Model file for the job. Use its own axes, mm. Face numbers are marked on the shaded views. A direction names the side the tool comes from. Round coordinates to 2 decimals unless told otherwise and drop trailing zeros. Loops run counter-clockwise (first coordinate to the right, second up) from the corner with the lowest first, then second, coordinate; pieces in that order, holes last. Notation, with made-up numbers: M 42.5,83.25 L 46.5,83.25 A10 ccw 46.5,100.25 Z; hole C 28,-11 d2. An arc over 180 degrees is marked long. Use a Markdown table: item, result. Add a question column.
Item 1: Two-plate mould, pull along Y, no slides. Class the marked faces 1, 2 and 3: +Y half, -Y half, draft (parallel to the pull), parting line (faces both ways), or undercut.
Item 2: Pin check, flat tips, straight feed: P1, Ø3, axis at y = -50, z = 10.5, coming from the +X side; P2, Ø1.5, axis at y = -76.5, z = 28, coming from the -X side; P3, Ø5, axis at y = 28, z = 74.5, coming from the +X side. Stop position of each tip, or through.
Item 3: Saw through at B-B on y = 164. Write the cut outline in (x, z), then the cut area to 3 significant figures.
Item 4: Tool access for the marked faces 4, 5 and 6: list every direction of +Z, -Z, +X, -X, +Y, -Y with a clear straight run to the whole face (end or side of a thin tool).
Item 5: Saw through at D-D on x = 133.5. Write the cut outline in (y, z), then the cut area to 3 significant figures.
Item 6: Saw through at A-A on z = -20. Write the cut outline in (x, y).
Item 7: Wall check: L1, parallel to X at y = -104.5, z = 5.5; L2, parallel to Z at x = 365, y = -188. Give the ranges that are in metal, low to high. Write a range as from..to.
Item 8: Saw through at C-C on x = -365.76. Write the cut outline in (y, z).
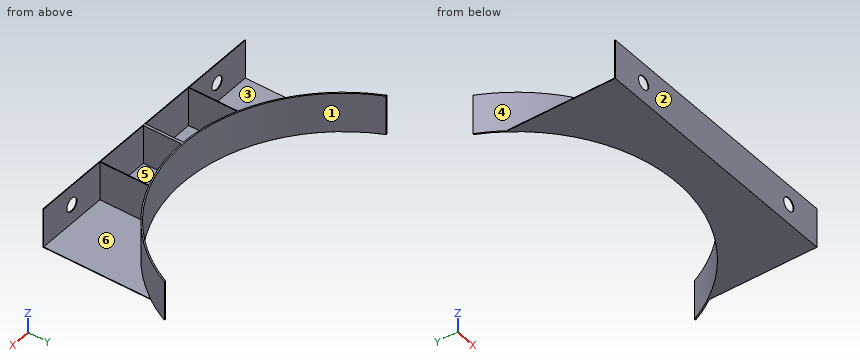
```python
from build123d import *

# Parameters (mm, degrees)
BOSS_EXTRUDE1_DEPTH = 6
BOSS_EXTRUDE2_DEPTH = 6
BOSS_EXTRUDE3_DEPTH = 0.1
SKETCH4_W           = 40
SKETCH4_H           = 6
BOSS_EXTRUDE4_DEPTH = 0.1
SKETCH7_R           = 1
CUT_EXTRUDE1_DEPTH  = 1.1
SCALE1_SCALE        = 25.4


with BuildPart() as part:
    # Sketch1 → Boss-Extrude1 (new body)
    with BuildSketch(Plane.XY):
        with BuildLine():
            Line((21.860143823, -10.193552473), (22.080622454, -10.193552473))
            ThreePointArc((22.080622454, -10.193552473), (0, -24.32), (-22.080622454, -10.193552473))
            Line((-22.080622454, -10.193552473), (-21.860143823, -10.193552473))
            ThreePointArc((-21.860143823, -10.193552473), (0, -24.12), (21.860143823, -10.193552473))
        make_face()
    extrude(amount=BOSS_EXTRUDE1_DEPTH)

    # Sketch2 → Boss-Extrude2 (add)
    with BuildSketch(Plane.XY):
        with BuildLine():
            Line((-0.2, -30.12), (0.2, -30.12))
            Line((0.2, -30.12), (0.2, -24.319177618))
            ThreePointArc((0.2, -24.319177618), (0, -24.32), (-0.2, -24.319177618))
            Line((-0.2, -24.319177618), (-0.2, -30.12))
        make_face()
        with BuildLine():
            Line((8.75, -30.12), (8.85, -30.12))
            Line((8.85, -30.12), (8.85, -22.652591463))
            ThreePointArc((8.85, -22.652591463), (8.8000214, -22.672053797), (8.75, -22.691405862))
            Line((8.75, -22.691405862), (8.75, -30.12))
        make_face()
        with BuildLine():
            Line((-8.75, -30.12), (-8.85, -30.12))
            Line((-8.85, -30.12), (-8.85, -22.652591463))
            ThreePointArc((-8.85, -22.652591463), (-8.8000214, -22.672053797), (-8.75, -22.691405862))
            Line((-8.75, -22.691405862), (-8.75, -30.12))
        make_face()
    extrude(amount=BOSS_EXTRUDE2_DEPTH)

    # Sketch3 → Boss-Extrude3 (add)
    with BuildSketch(Plane.XY):
        with BuildLine():
            Line((0, -30.12), (-20, -30.12))
            Line((-20, -30.12), (-20, -13.836993893))
            ThreePointArc((-20, -13.836993893), (0, -24.32), (20, -13.836993893))
            Line((20, -13.836993893), (20, -30.12))
            Line((20, -30.12), (0, -30.12))
        make_face()
    extrude(amount=BOSS_EXTRUDE3_DEPTH)

    # Sketch4 → Boss-Extrude4 (add)
    with BuildSketch(Plane(origin=(0, -30.12, 0), x_dir=(-1, 0, 0), z_dir=(0, -1, 0))):
        with Locations((0, -3)):
            Rectangle(SKETCH4_W, SKETCH4_H)
    extrude(amount=-BOSS_EXTRUDE4_DEPTH)

    # Sketch7 → Cut-Extrude1 (cut)
    with BuildSketch(Plane(origin=(0, -30.12, 0), x_dir=(-1, 0, 0), z_dir=(0, -1, 0))):
        with Locations((-14.4, -3)):
            Circle(SKETCH7_R)
        with Locations((14.4, -3)):
            Circle(SKETCH7_R)
    extrude(amount=-CUT_EXTRUDE1_DEPTH, mode=Mode.SUBTRACT)


with BuildPart() as part_1:
    # Scale1: scaled about (0, -23.561684395, 2.298462584)
    add(part.part.scale(SCALE1_SCALE).moved(Location((0, 574.905099238, -56.08248705))))


solid = part_1.part
```
Entries:
| question | item | result |
|---|---|---|
| 1 | face 1 | +Y half |
| 1 | face 2 | -Y half |
| 1 | face 3 | undercut |
| 2 | P1 | x = 224.79 |
| 2 | P2 | x = -224.79 |
| 2 | P3 | x = 291.91 |
| 3 | outline | M -508,-56.08 L -454.42,-56.08 L -454.42,96.32 L -461.24,96.32 L -461.24,-53.54 L -508,-53.54 Z; M 454.42,-56.08 L 508,-56.08 L 508,-53.54 L 461.24,-53.54 L 461.24,96.32 L 454.42,96.32 Z |
| 3 | area | 2,320 mm2 |
| 4 | face 4 | +Z, -X |
| 4 | face 5 | +Z |
| 4 | face 6 | +Z, +X |
| 5 | outline | M -190.14,-56.08 L -23.02,-56.08 L -23.02,96.32 L -28.22,96.32 L -28.22,-53.54 L -187.6,-53.54 L -187.6,96.32 L -190.14,96.32 Z |
| 5 | area | 1,590 mm2 |
| 6 | outline | M -560.85,315.99 A617.73 ccw -224.79,-0.47 L -224.79,-187.6 L -508,-187.6 L -508,-190.14 L 508,-190.14 L 508,-187.6 L 224.79,-187.6 L 224.79,-0.47 A617.73 ccw 560.85,315.99 L 555.25,315.99 A612.65 cw -555.25,315.99 Z; hole M -222.25,-187.6 L -5.08,-187.6 L -5.08,-42.8 A617.73 cw -222.25,-1.46 Z; hole M 5.08,-187.6 L 222.25,-187.6 L 222.25,-1.46 A617.73 cw 5.08,-42.8 Z |
| 7 | L1 | -224.79..-222.25, -5.08..5.08, 222.25..224.79 |
| 7 | L2 | -56.08..-5.27, 45.51..96.32 |
| 8 | outline | M -190.14,-56.08 L 83.42,-56.08 L 83.42,96.32 L 77.1,96.32 L 77.1,-53.54 L -187.6,-53.54 L -187.6,-5.28 L -190.14,-5.28 Z; M -190.14,45.52 L -187.6,45.52 L -187.6,96.32 L -190.14,96.32 Z |
